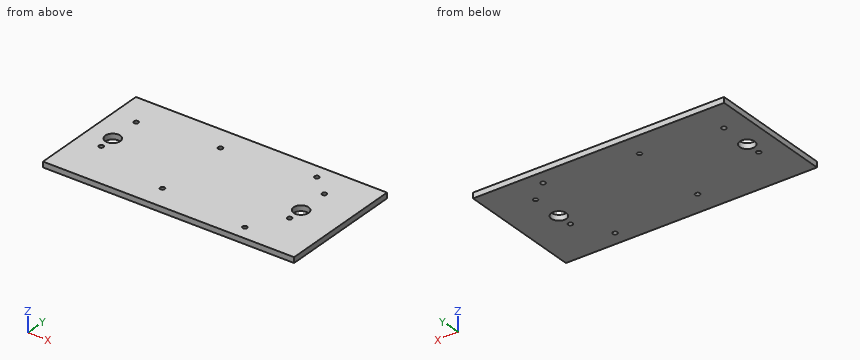
Autodesk Inventor part; units mm, degrees
ref_plane "YZ Plane" through (0, 0, 0) normal (1, 0, 0) x (0, 1, 0)
ref_plane "XZ Plane" through (0, 0, 0) normal (0, 1, 0) x (-1, 0, 0)
ref_plane "XY Plane" through (0, 0, 0) normal (0, 0, 1) x (1, 0, 0)
sketch "Sketch2" plane through (0, 0, 0) normal (0, 0, 1) x (1, 0, 0)
  line L0 (40, -40) -> (-70, -40)
  line L1 (-70, -40) -> (-70, 40)
  line L2 (-70, 40) -> (40, 40)
  circle A0 centre (-35, -25) radius 1
  circle A1 centre (-35, -25) radius 1.45
  circle A2 centre (22, -31) radius 1
  circle A3 centre (22, -31) radius 1.45
  circle A4 centre (22, 31) radius 1
  circle A5 centre (22, 31) radius 1.45
  circle A6 centre (-35, 25) radius 1
  circle A7 centre (-35, 25) radius 1.45
  line L3 (59.9998, -0.0003) -> (34.9998, -0.0003)
  line L4 (34.9998, -0.0003) -> (34.9998, -10.1033)
  line L5 (34.9998, -0.0003) -> (34.9998, 19.8967)
  circle A8 centre (34.9998, -10.1033) radius 1.45
  circle A9 centre (34.9998, 19.8967) radius 1.45
  line L6 (-60, 0) -> (-60, -10.103)
  line L7 (-60, -10.103) -> (-60, 0)
  line L8 (-60, 0) -> (-60, 19.897)
  circle A10 centre (-60, 19.897) radius 1.45
  circle A11 centre (-60, -10.103) radius 1.45
  line L9 (40, -40) -> (60, -40)
  line L10 (60, -40) -> (60, 40)
  line L11 (60, 40) -> (40, 40)
  line L12 (60, -40) -> (60, 0)
  line L13 (-70, 0) -> (-60, 0)
  point P0 (0, 0)
  dimension "d1" = 44.721
  dimension "d2" = 110
  dimension "d3" = 80
  dimension "d4" = 2.9
  dimension "d5" = 2.9
  dimension "d6" = 2.9
  dimension "d7" = 2.9
  dimension "d8" = 25
  dimension "d9" = 10.103
  dimension "d11" = 19.897
  dimension "d12" = 2.9
  dimension "d13" = 2.9
  dimension "d19" = 2.9
  dimension "d20" = 2.9
  dimension "d21" = 20
  dimension "d22" = 10
extrude "Extrusion1" add sketch "Sketch2" along normal blind 3.5 contours A10 | A11 | L0 L1 L2 L11 L10 L9
sketch "Sketch3" plane through (0, 0, 0) normal (0, 0, -1) x (-1, 0, 0)
  line L0 (70, 40) -> (70, -40)
  line L1 (70, 40) -> (100, 40)
  line L2 (100, 40) -> (100, -40)
  line L3 (100, -40) -> (70, -40)
  line L4 (70, -40) -> (70, 40)
  circle A0 centre (85, 19.9314) radius 1.45
  circle A1 centre (85, -10.0686) radius 1.45
  point P0 (0, 0)
  dimension "d23" = 30
  dimension "d25" = 2.9
  dimension "d26" = 2.9
extrude "Extrusion2" add sketch "Sketch3" against normal up to surface (3.5 mm away)
sketch "Sketch4" plane through (0, 0, 3.5) normal (0, 0, 1) x (1, 0, 0)
  circle A0 centre (34.9998, -10.1033) radius 1.45
  circle A1 centre (34.9998, -0.1713) radius 4.767
  circle A2 centre (-85, -10.0686) radius 1.45
  circle A3 centre (-85, -0.1713) radius 4.767
  point P0 (0, 0)
  dimension "d31" = 9.534
extrude "Extrusion3" cut sketch "Sketch4" against normal up to surface (3.5 mm away) contours A1 | A3
properties part number "lidar_plate"
The listing builds one solid part. Answer for the finished solid, in the listing's coordinates (mm). Coordinates: 2 decimals unless noted, no trailing zeros. Loops run counter-clockwise (first coordinate to the right, second up) from the corner with the lowest first, then second, coordinate; pieces in that order, holes last. Notation, with made-up numbers: (88, 27.5) - (129, 27.5) arc R23 ccw to (129, 41.5) - close; hole circle Ø4 at (78, 69). An arc over 180 degrees is marked (long way). Use a Markdown table: item, result. Add a question column.
1) The part is cut by section A-A, the plane x = -35. Give the vertices of the cut face in (y, z).
2) The part is cut by section C-C, the plane z = 1.25. State how many separate pieces and enclosed holes the cut face has, and give its area (3 significant figures).
3) Given pin 1 (4.5 mm diameter, centred on x = 35, y = 19.9, fed in from -Z); pin 2 (2.5 mm diameter, centred on x = 35, y = -10.1, fed in from -Z), each flat-ended and moving along its own axis, determine where each tip first touches the part or whether it passes through.
4) The part is cut by section B-B, the plane y = 31. Give the vertices of the cut face in (x, z), and give its area (3 significant figures).
5) Find the intervals of material crossed by line 1 (X direction, y = -10, z = 3.1); line 2 (Y direction, x = 22, z = 1.7); line 3 (Y direction, x = -85, z = 1.65), in increasing order.
Here are the results:
| question | item | result |
|---|---|---|
| 1 | outline | (-40, 0) - (-26.45, 0) - (-26.45, 3.5) - (-40, 3.5) - close; (-23.55, 0) - (23.55, 0) - (23.55, 3.5) - (-23.55, 3.5) - close; (26.45, 0) - (40, 0) - (40, 3.5) - (26.45, 3.5) - close |
| 2 | separate pieces | 1 |
| 2 | enclosed holes | 10 |
| 2 | area | 12,600 mm^2 |
| 3 | pin 1 | stops at z = 0 |
| 3 | pin 2 | passes through |
| 4 | outline | (-100, 0) - (20.55, 0) - (20.55, 3.5) - (-100, 3.5) - close; (23.45, 0) - (60, 0) - (60, 3.5) - (23.45, 3.5) - close |
| 4 | area | 550 mm^2 |
| 5 | line 1 | x = -100 to -86.45, -83.55 to 33.55, 36.45 to 60 |
| 5 | line 2 | y = -40 to -32.45, -29.55 to 29.55, 32.45 to 40 |
| 5 | line 3 | y = -40 to -11.52, -8.62 to -4.94, 4.6 to 18.48, 21.38 to 40 |
